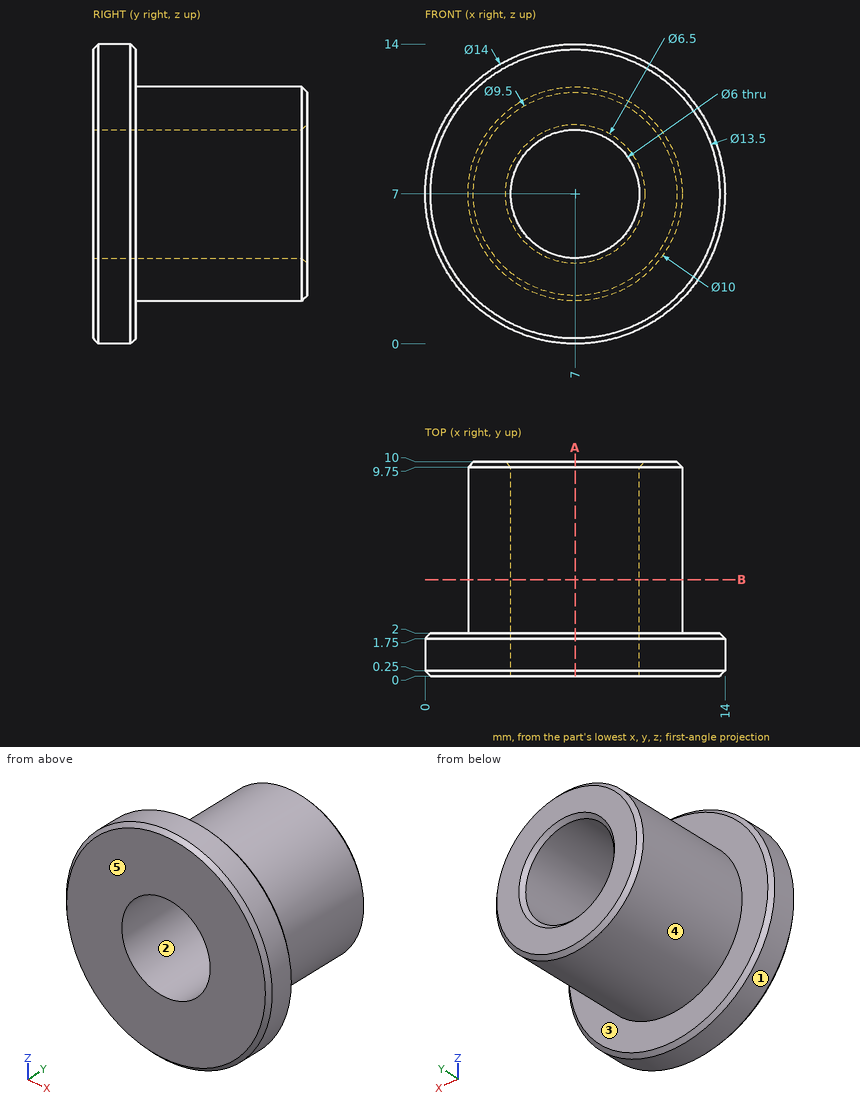
Geometry check sheet. Reference: drawing and pictorial views, mm from the part's lowest x, y, z. A direction names the side the tool comes from. Give positions to 0.01 mm unless a question says otherwise; leave off trailing zeros. Write each loop counter-clockwise with the first axis right and the second up, starting at its lowest first coordinate (ties: lowest second). Pieces come first, ordered by that corner, then holes.
Item 1: Gauge pin test, flat ends, axial feed: pin 1 (7 mm diameter, centred on x = 7, z = 7, fed in from +Y); pin 2 (1 mm diameter, centred on y = 3, z = 7.5, fed in from -X). Record the tip position at first contact, or that the pin passes through.
Item 2: Access from +Z, -Z, +X, -X, +Y, -Y to the whole of each face (thin tool, end or side, straight path). Record for the marked faces 4 and 5.
Item 3: Scan lines: L1, parallel to Z at x = 7, y = 4.75; L2, parallel to X at y = 5.25, z = 9.25. Record each from-to range of solid material in increasing order.
Item 4: Draft check along Z on the marked faces 1, 2 and 3. Enter one of: released by +Z, released by -Z, zero draft, split by the parting line, or undercut.
Item 5: Cross-section at A-A (x = 7). Enter the section's corners in (y, z).
Item 6: Cross-section at B-B (y = 4.5). Enter the section's corners in (x, z), and give its area (3 significant figures).
Report:
1. pin 1: stops at y = 10
1. pin 2: stops at x = 2
2. face 4: +Y
2. face 5: +Z, -Z, +X, -X, -Y
3. L1: z = 2 to 4, 10 to 12
3. L2: x = 2.53 to 5.02, 8.98 to 11.47
4. face 1: split by the parting line
4. face 2: undercut
4. face 3: zero draft
5. outline: (0, 0.25) - (0.25, 0) - (1.75, 0) - (2, 0.25) - (2, 2) - (9.75, 2) - (10, 2.25) - (10, 3.75) - (9.75, 4) - (0, 4) - close; (0, 10) - (9.75, 10) - (10, 10.25) - (10, 11.75) - (9.75, 12) - (2, 12) - (2, 13.75) - (1.75, 14) - (0.25, 14) - (0, 13.75) - close
6. outline: circle Ø10 at (7, 7); hole circle Ø6 at (7, 7)
6. area: 50.3 mm2
